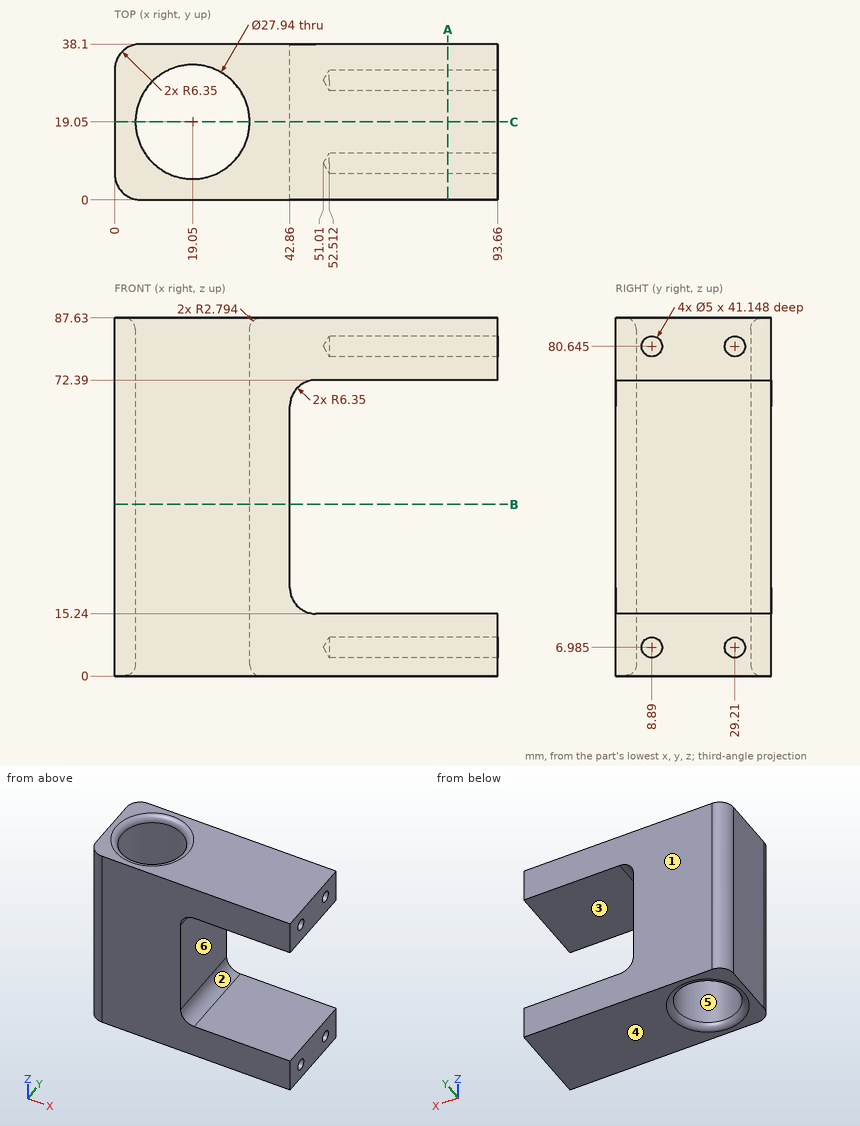
Geometry check sheet. Reference: drawing and pictorial views, mm from the part's lowest x, y, z. A direction names the side the tool comes from. Give positions to 0.01 mm unless a question says otherwise; leave off trailing zeros. Write each loop counter-clockwise with the first axis right and the second up, starting at its lowest first coordinate (ties: lowest second). Pieces come first, ordered by that corner, then holes. Notation, with made-up numbers: M -14,-11 L 26,-11 A28 ccw 26,13 Z; hole C -36,-33 d6. An arc over 180 degrees is marked long. Use CSV: the item, a comma, the result in double quotes.
1) Cross-section at B-B (z = 42). Enter the section's corners in (x, y).
Final values:
outline,"M 0,6.35 A6.35 ccw 6.35,0 L 42.86,0 L 42.86,38.1 L 6.35,38.1 A6.35 ccw 0,31.75 Z; hole C 19.05,19.05 d27.94"
2) Cross-section at C-C (y = 19.05). Enter the section's corners in (x, z), plus the area to 3 significant figures.
Final values:
outline,"M 0,0 L 2.29,0 A2.79 ccw 5.08,2.79 L 5.08,84.84 A2.79 ccw 2.29,87.63 L 0,87.63 Z; M 33.02,2.79 A2.79 ccw 35.81,0 L 93.66,0 L 93.66,15.24 L 49.21,15.24 A6.35 cw 42.86,21.59 L 42.86,66.04 A6.35 cw 49.21,72.39 L 93.66,72.39 L 93.66,87.63 L 35.81,87.63 A2.79 ccw 33.02,84.84 Z"
area,"2,870 mm²"
3) Access from +Z, -Z, +X, -X, +Y, -Y to the whole of each face (thin tool, end or side, straight path). Record for the marked faces 1 and 2.
Final values:
face 1,"+Z, -Z, +X, -X, +Y"
face 2,"+X, +Y, -Y"
4) Material ranges on line 1 along Y through (x, z) = (72.5, 7); line 2 along Z through (x, y) = (82, 3.5); line 3 along Y through (x, z) = (19.05, 48), recorded low to high.
Final values:
line 1,"0 to 6.39, 11.39 to 26.71, 31.71 to 38.1"
line 2,"0 to 15.24, 72.39 to 87.63"
line 3,"0 to 5.08, 33.02 to 38.1"
5) Go/stop test with flat-tipped pins: pin 1 Ø4 at (x, y) = (65, 18.5) entering from -Z; pin 2 Ø1 at (y, z) = (9, 65.5) entering from +X; pin 3 Ø4.5 at (y, z) = (29.21, 80.645) entering from +X; pin 4 Ø3 at (y, z) = (29.21, 6.985) entering from +X. Record where each tip stops, or that it passes through.
Final values:
pin 1,"z = 0"
pin 2,"x = 42.86"
pin 3,"x = 52.36"
pin 4,"x = 51.91"
6) Release check for a two-part mould opening along Z. For the marked faces 3, 4, 5 and 6 record: released by +Z, released by -Z, zero draft, split by the parting line, or undercut.
Final values:
face 3,"undercut"
face 4,"released by -Z"
face 5,"zero draft"
face 6,"undercut"
7) Cross-section at A-A (x = 81.5). Enter the section's corners in (y, z) (3 decimals).
Final values:
outline,"M 0,0 L 38.1,0 L 38.1,15.24 L 0,15.24 Z; M 0,72.39 L 38.1,72.39 L 38.1,87.63 L 0,87.63 Z; hole C 8.89,6.985 d5; hole C 8.89,80.645 d5; hole C 29.21,6.985 d5; hole C 29.21,80.645 d5"
